Geometry check sheet. Reference: drawing and pictorial views, mm from the part's lowest x, y, z. Give positions to 0.01 mm unless a question says otherwise; leave off trailing zeros. Order: outer loops, then holes, each group sorted by start corner. A loop starts at its lowest first (then second) coordinate and runs counter-clockwise, first axis right, second up.
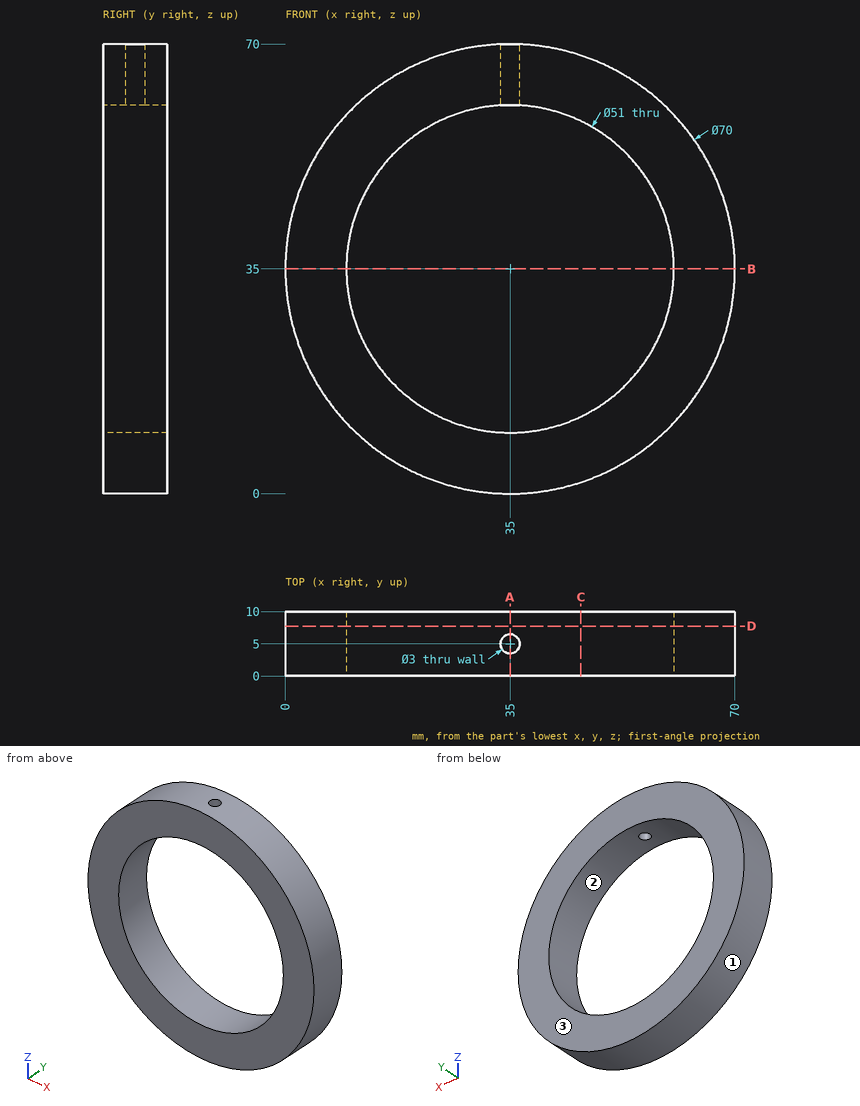
(1) Sectioned sample at B-B (z = 35). Enter the section's corners in (x, y), plus the area to 3 significant figures.
(2) Release check for a two-part mould opening along X. For the marked faces 1, 2 and 3 record: released by +X, released by -X, zero draft, split by the parting line, or undercut.
(3) Sectioned sample at A-A (x = 35). Enter the section's corners in (y, z).
(4) Go/stop test with flat-tipped pins: P1, Ø2, axis at y = 5.5, z = 48, coming from the -X side; P2, Ø5, axis at y = 2, z = 62.5, coming from the -X side; P3, Ø5, axis at x = 14, y = 7, coming from the +Z side. Record where each tip stops, or that it passes through.
(5) Thickness scan on L1, parallel to Z at x = 35, y = 2; L2, parallel to Y at x = 35, z = 67.25; L3, parallel to X at y = 5.5, z = 29.5. Record the ranges inside material, lowest first.
(6) Sectioned sample at C-C (x = 46). Enter the section's corners in (y, z), plus the area to 3 significant figures.
(7) Sectioned sample at D-D (y = 7.75). Enter the section's corners in (x, z).
Values follow:
1. outline: (0, 0) - (9.5, 0) - (9.5, 10) - (0, 10) - close; (60.5, 0) - (70, 0) - (70, 10) - (60.5, 10) - close
1. area: 190 mm2
2. face 1: split by the parting line
2. face 2: undercut
2. face 3: zero draft
3. outline: (0, 0) - (10, 0) - (10, 9.5) - (0, 9.5) - close; (0, 60.5) - (3.5, 60.5) - (3.5, 70) - (0, 70) - close; (6.5, 60.5) - (10, 60.5) - (10, 70) - (6.5, 70) - close
4. P1: stops at x = 2.12
4. P2: stops at x = 10.51
4. P3: stops at z = 64.71
5. L1: z = 0 to 9.5, 60.5 to 70
5. L2: y = 0 to 3.5, 6.5 to 10
5. L3: x = 0.43 to 10.1, 59.9 to 69.57
6. outline: (0, 1.77) - (10, 1.77) - (10, 11.99) - (0, 11.99) - close; (0, 58.01) - (10, 58.01) - (10, 68.23) - (0, 68.23) - close
6. area: 204 mm2
7. outline: circle Ø70 at (35, 35); hole circle Ø51 at (35, 35)
